Read the model definition and answer for the solid it produces. Units are mm, in the model's axes. Face numbers are marked on the shaded views. A direction names the side the tool comes from. Coordinates: 2 decimals unless noted, no trailing zeros. Order: outer loops, then holes, each group sorted by start corner. A loop starts at its lowest first (then second) coordinate and runs counter-clockwise, first axis right, second up. Notation, with made-up numbers: (68.25, 78.5) - (72.25, 78.5) arc R17 ccw to (72.25, 95.5) - close; hole circle Ø8 at (79.5, 71). An arc over 180 degrees is marked (long way). Answer as a JSON object with one key per item and string values. Group by question number.
from build123d import *

# Parameters (mm, degrees)
F0_R            = 47.625
F1_DEPTH        = 12.7
F2_R            = 19.812
F3_DEPTH        = 9.525
F4_R            = 22.987
F4_R_2          = 19.812
F5_DEPTH        = 3.175
F7_DEPTH        = 9.525
F9_DEPTH        = 1.5875
F9_COPIES_COUNT = 3


# Not quite as in the source:
# - a pattern or mirror of a feature is missing from the dataset's text; its kind, count and spacing are read off the source's solid


with BuildPart() as f1:
    # F0 (on Top) → F1 (new body)
    with BuildSketch(Plane.XY):
        Circle(F0_R)
    extrude(amount=F1_DEPTH)

    # F2 (on face) → F3 (join)
    with BuildSketch(Plane.XY.offset(12.7)):
        Circle(F2_R)
    extrude(amount=F3_DEPTH)

    # F4 (on face) → F5 (join)
    with BuildSketch(Plane.XY.offset(12.7)):
        Circle(F4_R)
        Circle(F4_R_2, mode=Mode.SUBTRACT)
    extrude(amount=F5_DEPTH)

    # F6 (on face) → F7 (cut, through all)
    with BuildSketch(Plane.XY.offset(22.225)):
        with BuildLine():
            Line((22.307688043, -5.5470012779), (20.3326952998, -4.406738686))
            ThreePointArc((20.3326952998, -4.406738686), (19.8803431182, -4.1693033149), (19.4103678781, -3.9690002312))
            ThreePointArc((19.4103678781, -3.9690002312), (17.1576952998, -9.906), (13.1424389669, -14.8253715637))
            ThreePointArc((13.1424389669, -14.8253715637), (13.5508941459, -15.1322305189), (13.9826952998, -15.405261314))
            Line((13.9826952998, -15.405261314), (15.957688043, -16.545523906))
            ThreePointArc((15.957688043, -16.545523906), (19.9073259568, -11.4935), (22.307688043, -5.5470012779))
        make_face()
        with BuildLine():
            ThreePointArc((13.1424389669, -14.8253715637), (17.1576952998, -9.906), (19.4103678781, -3.9690002312))
            ThreePointArc((19.4103678781, -3.9690002312), (11.6584339857, -6.731), (13.1424389669, -14.8253715637))
        make_face()
        with BuildLine():
            ThreePointArc((-13.9826952998, -15.405261314), (-13.5508941459, -15.1322305189), (-13.1424389669, -14.8253715637))
            ThreePointArc((-13.1424389669, -14.8253715637), (-17.1576952998, -9.906), (-19.4103678781, -3.9690002312))
            ThreePointArc((-19.4103678781, -3.9690002312), (-19.8803431182, -4.1693033149), (-20.3326952998, -4.406738686))
            Line((-20.3326952998, -4.406738686), (-22.307688043, -5.5470012779))
            ThreePointArc((-22.307688043, -5.5470012779), (-19.9073259568, -11.4935), (-15.957688043, -16.545523906))
            Line((-15.957688043, -16.545523906), (-13.9826952998, -15.405261314))
        make_face()
        with BuildLine():
            ThreePointArc((-19.4103678781, -3.9690002312), (-17.1576952998, -9.906), (-13.1424389669, -14.8253715637))
            ThreePointArc((-13.1424389669, -14.8253715637), (-11.6584339857, -6.731), (-19.4103678781, -3.9690002312))
        make_face()
        with BuildLine():
            ThreePointArc((-6.2679289112, 18.7943717949), (0, 13.462), (6.2679289112, 18.7943717949))
            ThreePointArc((6.2679289112, 18.7943717949), (0, 19.812), (-6.2679289112, 18.7943717949))
        make_face()
        with BuildLine():
            ThreePointArc((-6.2679289112, 18.7943717949), (0, 19.812), (6.2679289112, 18.7943717949))
            ThreePointArc((6.2679289112, 18.7943717949), (6.3294489723, 19.3015338338), (6.35, 19.812))
            Line((6.35, 19.812), (6.35, 22.0925251839))
            ThreePointArc((6.35, 22.0925251839), (0, 22.987), (-6.35, 22.0925251839))
            Line((-6.35, 22.0925251839), (-6.35, 19.812))
            ThreePointArc((-6.35, 19.812), (-6.3294489723, 19.3015338338), (-6.2679289112, 18.7943717949))
        make_face()
    extrude(amount=-F7_DEPTH, mode=Mode.SUBTRACT)

    # F8 (on Right) → F9 (join, symmetric)
    with BuildSketch(Plane.YZ):
        with BuildLine():
            Line((-21.5231496841, 11.5825022791), (-21.5231496841, 15.875))
            Line((-21.5231496841, 15.875), (-23.241, 15.875))
            Line((-23.241, 15.875), (-23.241, 17.5747702103))
            ThreePointArc((-23.241, 17.5747702103), (-23.8028498992, 19.2971673195), (-25.2722576527, 20.3569635098))
            Line((-25.2722576527, 20.3569635098), (-43.5602576527, 26.2054457308))
            ThreePointArc((-43.5602576527, 26.2054457308), (-46.1723971092, 25.7824025322), (-47.371, 23.4232524314))
            Line((-47.371, 23.4232524314), (-47.371, 11.5825022791))
            Line((-47.371, 11.5825022791), (-21.5231496841, 11.5825022791))
        make_face()
    f9 = extrude(amount=F9_DEPTH, both=True)

    # F9_copies: F9 ×3 about axis
    f9_copies_axis = Axis((0, 0, 0), (0, 0, 1))
    for i in range(1, F9_COPIES_COUNT):
        add(f9.rotate(f9_copies_axis, i * 360 / F9_COPIES_COUNT))


solid = f1.part
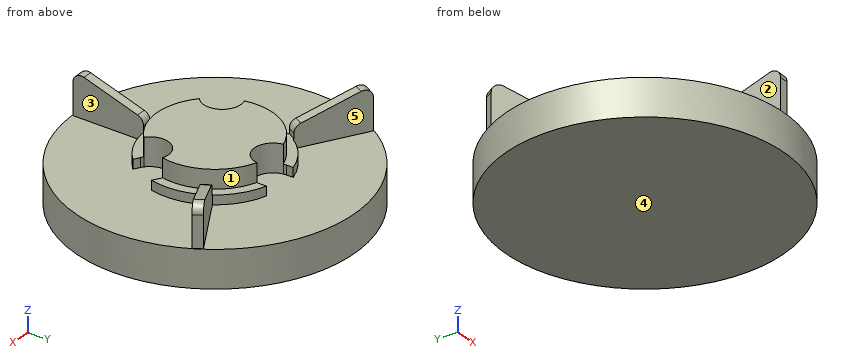
1. A cutting plane is placed at B-B on x = 0. Write down the section's boundary in (y, z) (3 decimals), and give its area (3 significant figures).
2. For the marked faces 4 and 5, determine the directions among +Z, -Z, +X, -X, +Y, -Y from which every point of the face is accessible in a straight line to the end or side of a thin tool.
3. A cutting plane is placed at C-C on y = 0. Write down the section's boundary in (x, z) (3 decimals).
4. Given pin 1 (4 mm diameter, centred on x = 33, z = 10.5, fed in from -Y); pin 2 (18.5 mm diameter, centred on x = 17.5, y = 9.5, fed in from +Z) (3 decimals); pin 3 (4 mm diameter, centred on y = -33.5, z = 21, fed in from +X); pin 4 (1.5 mm diameter, centred on x = 16.5, y = -1.5, fed in from -Z), each flat-ended and moving along its own axis, determine where each tip first touches the part or whether it passes through.
5. Straight lines are drawn through the part: L1, parallel to X at y = -9.5, z = 18.5; L2, parallel to Z at x = 41.5, y = 19.5; L3, parallel to Z at x = -2, y = -22.5 (3 decimals). For each, find the intervals that lie inside material, in ascending order.
6. For a pull along X with two mould halves and no side action, classify the marked faces 1, 2 and 3 as pulls with the +X half, pulls with the -X half, needs draft (parallel to the pull), parting line crosses it, or undercut.
7. A cutting plane is placed at A-A on z = 19. Write down the section's boundary in (x, y), and give its area (3 significant figures).
8. A cutting plane is placed at D-D on z = 7. Write down the section's boundary in (x, y) (3 decimals), and give its area (3 significant figures).
Derived:
{
 "1": {"outline": "(-47.625, 0) - (47.625, 0) - (47.625, 12.7) - (13.462, 12.7) - (13.462, 22.225) - (-19.812, 22.225) - (-19.812, 15.875) - (-23.241, 15.875) - (-23.241, 17.575) arc R2.921 ccw to (-25.272, 20.357) - (-43.56, 26.205) arc R2.921 ccw to (-47.371, 23.423) - (-47.371, 12.7) - (-47.625, 12.7) - close", "area": "1,800 mm2"},
 "2": {"face 4": "-Z, +X, -X, +Y, -Y", "face 5": "+Z, +Y"},
 "3": {"outline": "(-47.625, 0) - (47.625, 0) - (47.625, 12.7) - (22.987, 12.7) - (22.987, 15.875) - (19.812, 15.875) - (19.812, 22.225) - (-19.812, 22.225) - (-19.812, 15.875) - (-22.987, 15.875) - (-22.987, 12.7) - (-47.625, 12.7) - close"},
 "4": {"pin 1": "stops at y = -36.15", "pin 2": "stops at z = 22.225", "pin 3": "stops at x = 1.59", "pin 4": "stops at z = 0"},
 "5": {"L1": "x = -10.82 to 10.82", "L2": "z = 0 to 12.7", "L3": "z = 0 to 15.875"},
 "6": {"face 1": "undercut", "face 2": "pulls with the -X half", "face 3": "pulls with the +X half"},
 "7": {"outline": "(-41.82, 22.31) - (-21.24, 10.43) - (-19.66, 13.18) - (-40.23, 25.06) - close; (-19.41, -3.97) arc R6.35 cw to (-13.14, -14.83) arc R19.81 ccw to (13.14, -14.83) arc R6.35 cw to (19.41, -3.97) arc R19.81 ccw to (6.27, 18.79) arc R6.35 cw to (-6.27, 18.79) arc R19.81 ccw to start; (-1.59, -47.37) - (1.59, -47.37) - (1.59, -23.61) - (-1.59, -23.61) - close; (19.66, 13.18) - (21.24, 10.43) - (41.82, 22.31) - (40.23, 25.06) - close", "area": "1,280 mm2"},
 "8": {"outline": "circle Ø95.25 at (0, 0)", "area": "7,130 mm2"}
}
